The model under review builds one solid part; all positions refer to its coordinate system, in mm. A direction names the side the tool comes from. Give positions to 0.01 mm unless a question says otherwise; leave off trailing zeros. Loops run counter-clockwise (first coordinate to the right, second up) from the corner with the lowest first, then second, coordinate; pieces in that order, holes last. Notation, with made-up numbers: (0.5, 87.5) - (58.5, 87.5) arc R17 cw to (58.5, 109.5) - close; hole circle Ø8 at (65, -2). An arc over 180 degrees is marked (long way). Return JSON: item names as keys, results as strings. Group by question number.
from build123d import *

# Parameters (mm, degrees)
F1_DEPTH = 6
F2_R     = 5
F3_W     = 50
F3_H     = 5.87
F4_DEPTH = 25


with BuildPart() as f1:
    # F0 (on Top) → F1 (new body)
    with BuildSketch(Plane.XY):
        with BuildLine():
            ThreePointArc((170.193543, -19.389994), (173.797456, -18.835445), (177.068441, -17.224121))
            ThreePointArc((177.068441, -17.224121), (210.314706, 23.380525), (213.658845, 75.752924))
            ThreePointArc((213.658845, 75.752924), (200.483313, 115.151894), (182.680857, 152.687823))
            ThreePointArc((182.680857, 152.687823), (134.513109, 160.754816), (86.985857, 171.996198))
            ThreePointArc((86.985857, 171.996198), (44.36332, 177.732663), (2.913726, 166.264491))
            ThreePointArc((2.913726, 166.264491), (-76.082674, 115.030345), (-126.918851, 35.777256))
            ThreePointArc((-126.918851, 35.777256), (-122.637212, -0.376763), (-91.614817, -19.430806))
            Line((-91.614817, -19.430806), (-86.660196, -19.485899))
            Line((-86.660196, -19.485899), (-86.660196, -13.485899))
            Line((-86.660196, -13.485899), (-76.660196, -13.485899))
            Line((-76.660196, -13.485899), (-76.660196, -18.485899))
            ThreePointArc((-76.660196, -18.485899), (-76.367303, -19.193006), (-75.660196, -19.485899))
            Line((-75.660196, -19.485899), (-67.660196, -19.485899))
            ThreePointArc((-67.660196, -19.485899), (-66.953089, -19.193006), (-66.660196, -18.485899))
            Line((-66.660196, -18.485899), (-66.660196, -13.485899))
            Line((-66.660196, -13.485899), (-31.660196, -13.485899))
            Line((-31.660196, -13.485899), (-31.660196, -18.485899))
            ThreePointArc((-31.660196, -18.485899), (-31.367303, -19.193006), (-30.660196, -19.485899))
            Line((-30.660196, -19.485899), (17.339804, -19.485899))
            ThreePointArc((17.339804, -19.485899), (18.046911, -19.193006), (18.339804, -18.485899))
            Line((18.339804, -18.485899), (18.339804, -13.485899))
            Line((18.339804, -13.485899), (18.339804, 28.364893))
            Line((18.339804, 28.364893), (-41.863095, 28.364893))
            Line((-41.863095, 28.364893), (-41.863095, 108.756206))
            Line((-41.863095, 108.756206), (169.688459, 108.756206))
            Line((169.688459, 108.756206), (169.688459, 28.364893))
            Line((169.688459, 28.364893), (132.439804, 28.364893))
            Line((132.439804, 28.364893), (132.439804, -13.485899))
            Line((132.439804, -13.485899), (132.439804, -17.485899))
            ThreePointArc((132.439804, -17.485899), (133.02559, -18.900112), (134.439804, -19.485899))
            Line((134.439804, -19.485899), (156.439804, -19.485899))
            ThreePointArc((156.439804, -19.485899), (157.146911, -19.193006), (157.439804, -18.485899))
            Line((157.439804, -18.485899), (157.439804, -13.485899))
            Line((157.439804, -13.485899), (167.439804, -13.485899))
            Line((167.439804, -13.485899), (167.439804, -18.450465))
            ThreePointArc((167.439804, -18.450465), (167.745112, -19.169773), (168.47461, -19.44986))
            Line((168.47461, -19.44986), (170.193543, -19.389994))
        make_face()
    extrude(amount=F1_DEPTH)

    # F2
    f2_edges = [f1.edges().sort_by_distance(p)[0] for p in [
        (-41.863095, 108.756206, 3),
        (-41.863095, 28.364893, 3),
        (18.339804, 28.364893, 3),
        (169.688459, 108.756206, 3),
        (169.688459, 28.364893, 3),
        (132.439804, 28.364893, 3),
    ]]
    fillet(f2_edges, radius=F2_R)

    # F3 (on face) → F4 (cut)
    with BuildSketch(Plane.XY.offset(6)):
        Polygon((-88.078382, 91.432652), (-113.348544, 48.288487), (-108.283419, 45.32177), (-83.013257, 88.465935), align=None)
        with Locations((60.208148, 166.061319)):
            Rectangle(F3_W, F3_H)
        Polygon((172.10519, 148.548136), (122.972107, 157.818528), (121.883763, 152.050304), (171.016846, 142.779912), align=None)
        Polygon((205.997825, 86.744264), (185.293966, 132.256353), (179.950847, 129.82572), (200.654705, 84.313631), align=None)
        Polygon((175.953445, -4.115971), (181.050032, -7.028307), (205.856984, 36.383847), (200.760397, 39.296184), align=None)
    extrude(amount=-F4_DEPTH, mode=Mode.SUBTRACT)


solid = f1.part
Item 1: For P1, Ø2, axis at x = -20, z = 2, coming from the +Y side; P2, Ø2, axis at x = -71.5, z = 3, coming from the +Y side; P3, Ø3, axis at x = 153, z = 4.5, coming from the +Y side, all flat-tipped, find the tip position at first contact; note any pin that passes through.
Item 2: Take a section at B-B (y = 59). State the section outline as (x, z) points.
Item 3: Take a section at C-C (z = 1). State how many separate pieces and enclosed holes the cut face has, then the cut area to 3 significant figures.
Item 4: Take a section at A-A (y = 124). State the section outline as (x, z) points, then the cut area to 3 significant figures.
Item 5: For L1, parallel to X at y = 96.5, z = 5.25; L2, parallel to X at y = 22.5, z = 4; L3, parallel to Y at x = 3, z = 2.5, list the stretches that pass through material, from the lowest coordinate up. Write a range as from..to.
Item 6: Mouldability with a two-part tool opening along Y and no side actions: class faces 4 (the face through (63, 108.756, 3)), 5 (the face through (-82, -13.486, 3)), 6 (the face through (190.158, 107.388, 3.042)), 7 (the face through (18.34, 2, 3)) as +Y half, -Y half, draft (parallel to the pull), parting line (faces both ways), or undercut.
Item 7: Tool access review of faces 1 (the face through (132.44, 3, 3)), 2 (the face through (210.04, 22.69, 2.96)), 3 (the face through (188.53, 17.89, 3.04)): name each direction out of +Z, -Z, +X, -X, +Y, -Y from which nothing blocks a thin tool from reaching the whole face with its end or side.
Item 8: Take a section at D-D (x = 113). State the section outline as (y, z) points, then the cut area to 3 significant figures.
Check sheet entries:
{
 "1": {"P1": "stops at y = 156.57", "P2": "stops at y = 120.45", "P3": "stops at y = 157.53"},
 "2": {"outline": "(-116.7, 0) - (-107.07, 0) - (-107.07, 6) - (-116.7, 6) - close; (-100.27, 0) - (-41.86, 0) - (-41.86, 6) - (-100.27, 6) - close; (169.69, 0) - (216.16, 0) - (216.16, 6) - (169.69, 6) - close"},
 "3": {"separate pieces": "1", "enclosed holes": "5", "area": "30,800 mm^2"},
 "4": {"outline": "(-66.62, 0) - (182.6, 0) - (182.6, 6) - (-66.62, 6) - close; (189.05, 0) - (196.78, 0) - (196.78, 6) - (189.05, 6) - close", "area": "1,540 mm^2"},
 "5": {"L1": "x = -92.58..-41.86, 169.69..195.11, 201.56..207.38", "L2": "x = -129.21..18.34, 132.44..191.16, 197.92..209.96", "L3": "y = -19.49..28.36, 108.76..166.31"},
 "6": {"face 4": "undercut", "face 5": "-Y half", "face 6": "undercut", "face 7": "draft"},
 "7": {"face 1": "+Z, -Z, -Y", "face 2": "+Z, -Z, +X", "face 3": "+Z, -Z"},
 "8": {"outline": "(108.76, 0) - (165.43, 0) - (165.43, 6) - (108.76, 6) - close", "area": "340 mm^2"}
}
